Design review of the part built by this model. Coordinates are the model's own, in mm. A direction names the side the tool comes from. Round coordinates to 2 decimals unless told otherwise and drop trailing zeros. Loops run counter-clockwise (first coordinate to the right, second up) from the corner with the lowest first, then second, coordinate; pieces in that order, holes last. Notation, with made-up numbers: M 52,72 L 78,72 A30 ccw 78,97 Z; hole C 62.5,43 d7. An arc over 180 degrees is marked long. One line per item, written item: value. Start each with the question number.
Item 1: For faces 1 (the flat face through (493, 12, 4.2)), 2 (the flat face through (493, 24.664, 14)), 3 (the flat face through (493, 26.264, 15)), list the 3-axis set-ups (+Z, -Z, +X, -X, +Y, -Y) from which the entire face can be reached by the end or side of a thin tool; tool diameter is ignored.
Item 2: Clearance check with a flat-ended pin moving along its axis: pin 1 (1.3 mm diameter, centred on x = 702, z = 0.5, fed in from +Y). State where the tip first meets the part, or that it passes through.
Item 3: We need section A-A (y = 11.5). Write out the cut boundary in (x, z).
Item 4: We need section B-B (z = 11.75). Write out the cut boundary in (x, y).
Item 5: Mouldability with a two-part tool opening along Z and no side actions: class faces 4 (the flat face through (493, 1.6, 14)), 5 (the flat face through (493, 13, 26.264)), 6 (the flat face through (0, 13, 3)) as released by +Z, released by -Z, zero draft, split by the parting line, or undercut.
Item 6: We need section C-C (x = 318). Write out the cut boundary in (y, z) (3 decimals), then the cut area to 3 significant figures.
Item 7: For line 1 along Z through (x, y) = (202.5, 18.5) (3 decimals); line 2 along Y through (x, z) = (129, 9.75); line 3 along Z through (x, y) = (678, 8), list the stretches that pass through material, from the lowest coordinate up.
from build123d import *

# Parameters (mm, degrees)
F1_DEPTH = 1000


with BuildPart() as f1:
    # F0 (on Right) → F1 (new body)
    with BuildSketch(Plane.YZ):
        with BuildLine():
            ThreePointArc((26.264214, 25.964214), (26.176346, 26.176346), (25.964214, 26.264214))
            Line((25.964214, 26.264214), (0.3, 26.264214))
            ThreePointArc((0.3, 26.264214), (0.087868, 26.176346), (0, 25.964214))
            Line((0, 25.964214), (0, 0.3))
            ThreePointArc((0, 0.3), (0.087868, 0.087868), (0.3, 0))
            Line((0.3, 0), (22, 0))
            Line((22, 0), (22, 1.575))
            Line((22, 1.575), (17, 1.575))
            Line((17, 1.575), (17, 2.625))
            Line((17, 2.625), (22, 2.625))
            Line((22, 2.625), (22, 4.2))
            Line((22, 4.2), (1.9, 4.2))
            ThreePointArc((1.9, 4.2), (1.687868, 4.287868), (1.6, 4.5))
            Line((1.6, 4.5), (1.6, 24.364214))
            ThreePointArc((1.6, 24.364214), (1.687868, 24.576346), (1.9, 24.664214))
            Line((1.9, 24.664214), (24.364214, 24.664214))
            ThreePointArc((24.364214, 24.664214), (24.576346, 24.576346), (24.664214, 24.364214))
            Line((24.664214, 24.364214), (24.664214, 4.264214))
            Line((24.664214, 4.264214), (25.964214, 4.264214))
            ThreePointArc((25.964214, 4.264214), (26.176346, 4.352082), (26.264214, 4.564214))
            Line((26.264214, 4.564214), (26.264214, 25.964214))
        make_face()
    extrude(amount=F1_DEPTH)


solid = f1.part
A:
1. face 1: +X, -X
1. face 2: -Z, +X, -X
1. face 3: +Z, -Z, +X, -X, +Y
2. pin 1: y = 22
3. outline: M 0,0 L 1000,0 L 1000,4.2 L 0,4.2 Z; M 0,24.66 L 1000,24.66 L 1000,26.26 L 0,26.26 Z
4. outline: M 0,0 L 1000,0 L 1000,1.6 L 0,1.6 Z; M 0,24.66 L 1000,24.66 L 1000,26.26 L 0,26.26 Z
5. face 4: undercut
5. face 5: released by +Z
5. face 6: zero draft
6. outline: M 0,0.3 A0.3 ccw 0.3,0 L 22,0 L 22,1.575 L 17,1.575 L 17,2.625 L 22,2.625 L 22,4.2 L 1.9,4.2 A0.3 cw 1.6,4.5 L 1.6,24.364 A0.3 cw 1.9,24.664 L 24.364,24.664 A0.3 cw 24.664,24.364 L 24.664,4.264 L 25.964,4.264 A0.3 ccw 26.264,4.564 L 26.264,25.964 A0.3 ccw 25.964,26.264 L 0.3,26.264 A0.3 ccw 0,25.964 Z
6. area: 195 mm2
7. line 1: 0 to 1.575, 2.625 to 4.2, 24.664 to 26.264
7. line 2: 0 to 1.6, 24.66 to 26.26
7. line 3: 0 to 4.2, 24.66 to 26.26
